Part model, mm, in its own coordinate system. Round coordinates to 2 decimals unless told otherwise and drop trailing zeros. Write each loop counter-clockwise with the first axis right and the second up, starting at its lowest first coordinate (ties: lowest second). Pieces come first, ordered by that corner, then holes. Notation, with made-up numbers: (18, 42) -> (46, 42) arc R8 cw to (46, 55) -> close; hole circle Ø9 at (39, 36). An arc over 180 degrees is marked (long way). Use CSV: the item, a comma, the result in double quotes. Start each with the question number.
(1) Saw through at A-A (y = -5.25). Give the cut face in (x, z), plus the area to 3 significant figures.
(2) Probe line 1 (X direction, y = -1.5, z = 239); line 2 (X direction, y = -8.4, z = 5); line 3 (Z direction, x = 4, y = -9.25). List the from-to ranges inside material, lowest first. Write a range as [from, to].
(3) Saw through at B-B (z = 112). Give the cut face in (x, y).
(4) Drop a flat-ended pin along its axis: pin 1 (2 mm diameter, centred on x = 4, z = 205, fed in from +Y). Give the stop position or say it passes through.
```python
from build123d import *

# Parameters (mm, degrees)
BOSS_EXTRU_1_DEPTH      = 260
ESQUISSE2_R             = 1.25
ENL_V_MAT_EXTRU_1_DEPTH = 10
ESQUISSE3_R             = 1.25
ENL_V_MAT_EXTRU_2_DEPTH = 10


with BuildPart() as part:
    # Esquisse1 → Boss.-Extru.1 (new body)
    with BuildSketch(Plane.XY):
        Polygon((0, 0), (0, -10), (10, -10), (10, 0), (8, 0), (8, -8), (2, -8), (2, 0), align=None)
    extrude(amount=BOSS_EXTRU_1_DEPTH)

    # Esquisse2 → Enlèv. mat.-Extru.1 (cut)
    with BuildSketch(Plane.XZ.offset(10)):
        with Locations(Location((5, 214.21, 0), (0, 0, 270))):
            Circle(ESQUISSE2_R)
    extrude(amount=-ENL_V_MAT_EXTRU_1_DEPTH, mode=Mode.SUBTRACT)

    # Esquisse3 → Enlèv. mat.-Extru.2 (cut)
    with BuildSketch(Plane(origin=(0, -10, 0), x_dir=(-1, 0, 0), z_dir=(0, -1, 0))):
        with Locations(Location((-5, -5, 0), (0, 0, 90))):
            Circle(ESQUISSE3_R)
        with Locations(Location((-5, -55, 0), (0, 0, 90))):
            Circle(ESQUISSE3_R)
    extrude(amount=-ENL_V_MAT_EXTRU_2_DEPTH, mode=Mode.SUBTRACT)


solid = part.part
```
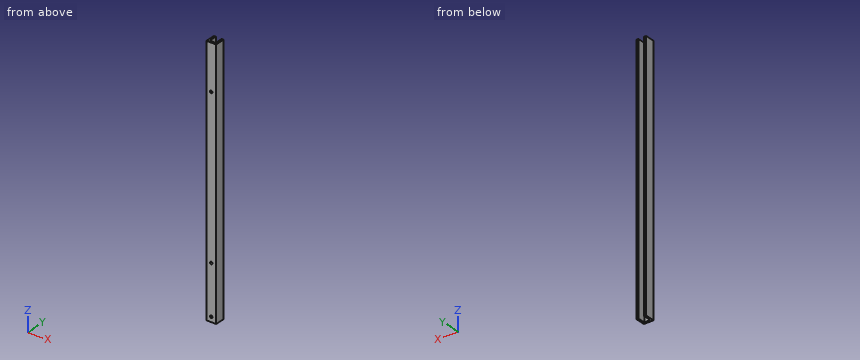
Answers:
1,outline,"(0, 0) -> (2, 0) -> (2, 260) -> (0, 260) -> close; (8, 0) -> (10, 0) -> (10, 260) -> (8, 260) -> close"
1,area,"1,040 mm²"
2,line 1,"x = [0, 2], [8, 10]"
2,line 2,"x = [0, 3.75], [6.25, 10]"
2,line 3,"z = [0, 4.25], [5.75, 54.25], [55.75, 213.46], [214.96, 260]"
3,outline,"(0, -10) -> (10, -10) -> (10, 0) -> (8, 0) -> (8, -8) -> (2, -8) -> (2, 0) -> (0, 0) -> close"
4,pin 1,"stops at y = -8"
